```python
from build123d import *

# Parameters (mm, degrees)
SKETCH1_W       = 6
SKETCH1_H       = 12
EXTRUDE1_DEPTH  = 6
SKETCH3_W       = 4
SKETCH3_H       = 8.6
EXTRUDE2_DEPTH  = 1
SKETCH2_R       = 1.25
EXTRUDE3_DEPTH  = 5.5
EXTRUDE4_DEPTH  = 4
SKETCH6_R       = 3
EXTRUDE5_DEPTH  = 1
SKETCH7_R       = 1.25
EXTRUDE6_DEPTH  = 4
SKETCH8_R       = 2.5
EXTRUDE7_DEPTH  = 3
FILLET1_R       = 4
EXTRUDE9_START  = -4
EXTRUDE9_DEPTH  = 4
EXTRUDE10_DEPTH = 2
SKETCH14_R      = 1.25
EXTRUDE11_DEPTH = 4


with BuildPart() as part:
    # Sketch1 → Extrude1 (new body)
    with BuildSketch(Plane.XY):
        with Locations((-1, 0)):
            Rectangle(SKETCH1_W, SKETCH1_H)
    extrude(amount=EXTRUDE1_DEPTH)

    # Sketch3 → Extrude2 (add)
    with BuildSketch(Plane.XY.offset(6)):
        Rectangle(SKETCH3_W, SKETCH3_H)
    extrude(amount=EXTRUDE2_DEPTH)

    # Sketch2 → Extrude3 (cut)
    with BuildSketch(Plane(origin=(0, 0, 0), x_dir=(-1, 0, 0), z_dir=(0, 0, -1))):
        with Locations((1, 3)):
            Circle(SKETCH2_R)
        with Locations((1, -3)):
            Circle(SKETCH2_R)
    extrude(amount=-EXTRUDE3_DEPTH, mode=Mode.SUBTRACT)

    # Sketch4 → Extrude4 (add)
    with BuildSketch(Plane(origin=(2, 0, 0), x_dir=(0, 0, -1), z_dir=(1, 0, 0))):
        with BuildLine():
            Line((-9.708497378, 6), (-6, 6))
            Line((-6, 6), (-6, -6))
            Line((-6, -6), (-9.708497378, -6))
            ThreePointArc((-9.708497378, -6), (-23, 0), (-9.708497378, 6))
        make_face()
    extrude(amount=-EXTRUDE4_DEPTH)

    # Sketch6 → Extrude5 (cut)
    with BuildSketch(Plane.ZY.offset(2)):
        with Locations(Location((15, 0, 0), (0, 0, 270))):
            Circle(SKETCH6_R)
    extrude(amount=-EXTRUDE5_DEPTH, mode=Mode.SUBTRACT)

    # Sketch7 → Extrude6 (cut)
    with BuildSketch(Plane.ZY.offset(2)):
        with Locations(Location((15, -5, 0), (0, 0, 270))):
            Circle(SKETCH7_R)
        with Locations(Location((15, 5, 0), (0, 0, 270))):
            Circle(SKETCH7_R)
    extrude(amount=-EXTRUDE6_DEPTH, mode=Mode.SUBTRACT)

    # Sketch8 → Extrude7 (cut)
    with BuildSketch(Plane.ZY.offset(1)):
        with Locations(Location((15, 0, 0), (0, 0, 270))):
            Circle(SKETCH8_R)
    extrude(amount=-EXTRUDE7_DEPTH, mode=Mode.SUBTRACT)

    # Fillet1
    fillet1_edges = [part.edges().sort_by_distance(p)[0] for p in [
        (0, -6, 9.708497378),
        (0, 6, 9.708497378),
    ]]
    fillet(fillet1_edges, radius=FILLET1_R)

    # Sketch12 → Extrude9 (add)
    with BuildSketch(Plane.ZY.offset(2).offset(EXTRUDE9_START)):
        with BuildLine():
            Line((16.582575695, -7.841903734), (23.510778925, -11.841903734))
            Line((23.510778925, -11.841903734), (29.510778925, -1.449598888))
            Line((29.510778925, -1.449598888), (22.582575695, 2.550401112))
            ThreePointArc((22.582575695, 2.550401112), (21.92820323, -4), (16.582575695, -7.841903734))
        make_face()
    extrude(amount=EXTRUDE9_DEPTH)

    # Sketch13 → Extrude10 (add)
    with BuildSketch(Plane.ZY.offset(2)):
        Polygon((29.510778925, -1.449598888), (25.613664608, 0.800401112), (19.613664608, -9.591903734), (23.510778925, -11.841903734), align=None)
    extrude(amount=EXTRUDE10_DEPTH)

    # Sketch14 → Extrude11 (cut)
    with BuildSketch(Plane(origin=(0, -13.140941839, 22.760778925), x_dir=(1, 0, 0), z_dir=(0, -0.5000000000000007, 0.8660254037844383))):
        with Locations(Location((-1, 4.5, 0), (0, 0, 270))):
            Circle(SKETCH14_R)
        with Locations(Location((-1, 10.5, 0), (0, 0, 270))):
            Circle(SKETCH14_R)
    extrude(amount=-EXTRUDE11_DEPTH, mode=Mode.SUBTRACT)


solid = part.part
```
CAD build for the part. Positions are in the model's coordinates, mm. A direction names the side the tool comes from. Give positions to 0.01 mm unless a question says otherwise; leave off trailing zeros. Order: outer loops, then holes, each group sorted by start corner. A loop starts at its lowest first (then second) coordinate and runs counter-clockwise, first axis right, second up.
(1) Saw through at D-D, the plane y = 5. Give the cut face in (x, z) (3 decimals).
(2) Tool access for faces 5 (the cylindrical face through (-0.079, 3.845, 2.712)), 6 (the flat face through (-2, -3, 13)), 7 (the flat face through (-3, 0, 6)), 8 (the cylindrical face through (-1.51, 0.65, 12.07)): list every direction of +Z, -Z, +X, -X, +Y, -Y with a clear straight run to the whole face (end or side of a thin tool).
(3) Saw through at A-A, the plane x = 1.65. Give the cut face in (y, z), then the cut area to 3 significant figures.
(4) Drill centre lines: L1, parallel to Y at x = -1, z = 2.6; L2, parallel to Y at x = 0.6, z = 6.25; L3, parallel to X at y = -3.5, z = 22.5. Where is each one in solid material? Low to high.
(5) Mould opens along Y. For faces 1 (the flat face through (2, 0, 11)), 2 (the flat face through (-0.982, -2.033, 24.555)), 3 (the flat face through (-0.96, -6.72, 26.47)), 4 (the flat face through (-2.986, -4.323, 22.656)) say: released by +Y, released by -Y, zero draft, split by the parting line, or undercut.
(6) Saw through at B-B, the plane y = 0. Give the cut face in (x, z), then the cut area to 3 significant figures.
(7) Saw through at C-C, the plane z = 5. Give the cut face in (x, y).
(8) Flat gauge pins, fed straight in: pin 1 (3 mm diameter, centred on x = 1, z = 10.5, fed in from +Y); pin 2 (2 mm diameter, centred on x = -1, y = 3, fed in from -Z); pin 3 (3 mm diameter, centred on x = -0.5, y = 3, fed in from -Z); pin 4 (3 mm diameter, centred on y = -5, z = 15, fed in from -X). Where does each tip first touch, or does it go through?
Results found:
1. outline: (-4, 0) - (2, 0) - (2, 13.75) - (-2, 13.75) - (-2, 6) - (-4, 6) - close; (-2, 16.25) - (2, 16.25) - (2, 21.245) - (-2, 21.245) - close
2. face 5: -Z
2. face 6: -X, +Y
2. face 7: -X, +Y, -Y
2. face 8: -X
3. outline: (-11.84, 23.51) - (-7.84, 16.58) arc R8 ccw to (-6.67, 10.58) arc R4 cw to (-6, 8.37) - (-6, 0) - (6, 0) - (6, 8.37) arc R4 cw to (6.67, 10.58) arc R8 ccw to (2.55, 22.58) - (-1.45, 29.51) - close; hole circle Ø2.5 at (-5, 15); hole circle Ø5 at (0, 15); hole circle Ø2.5 at (5, 15)
3. area: 339 mm2
4. L1: y = -6 to -4.25, -1.75 to 1.75, 4.25 to 6
4. L2: y = -6 to 6
4. L3: x = -2 to 2
5. face 1: zero draft
5. face 2: undercut
5. face 3: released by -Y
5. face 4: released by +Y
6. outline: (-4, 0) - (2, 0) - (2, 12.5) - (-1, 12.5) - (-1, 12) - (-2, 12) - (-2, 6) - (-4, 6) - close; (-4, 25.15) - (-2, 25.15) - (-2, 18) - (-1, 18) - (-1, 17.5) - (2, 17.5) - (2, 27) - (-4, 27) - close
6. area: 103 mm2
7. outline: (-4, -6) - (2, -6) - (2, 6) - (-4, 6) - close; hole circle Ø2.5 at (-1, -3); hole circle Ø2.5 at (-1, 3)
8. pin 1: stops at y = 7.42
8. pin 2: stops at z = 5.5
8. pin 3: stops at z = 0
8. pin 4: stops at x = -2
